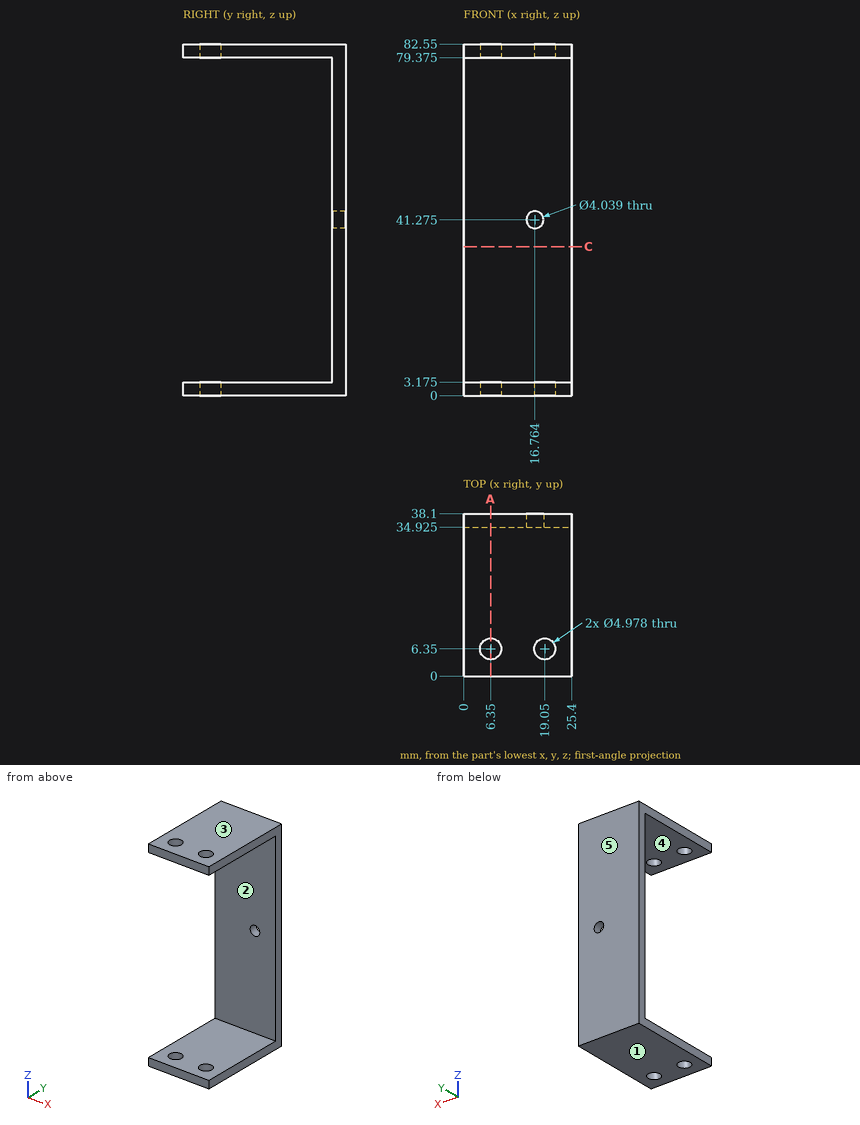
Can you work these out from the drawing? Everything is in mm from the part's minimum corner. A direction names the side the tool comes from. Round coordinates to 2 decimals unless told otherwise and drop trailing zeros. Loops run counter-clockwise (first coordinate to the right, second up) from the corner with the lowest first, then second, coordinate; pieces in that order, holes last. Notation, with made-up numbers: (-24, -19.75) - (19, -19.75) arc R20 cw to (19, 0.25) - close; hole circle Ø8 at (49, 13). An arc over 180 degrees is marked (long way). Write item = value, one per line. Start each with the question number.
(1) If we mould it in two halves opening along Z, with no side actions, what happens to the marked faces 3, 4 and 5? For each: released by +Z, released by -Z, zero draft, split by the parting line, or undercut.
(2) If we section it at C-C (z = 35): Please give me the cut outline in (x, y) (1 decimal).
(3) If we section it at A-A (x = 6.35): Give the number of separate pieces and of enclosed holes in the cut face.
(4) If I drill on probe 1 along X at (y, z) = (6, 80) (1 decimal); probe 2 along Y at (x, z) = (19.05, 81.2); probe 3 along Y at (x, z) = (10, 70) (1 decimal), over which ranges is the centre line in solid material (lowest first)? Write a range as [from, to].
(5) For the marked faces 1 and 2, which set-ups out of +Z, -Z, +X, -X, +Y, -Y let a thin tool reach every point of the face, with its end or its side?
(6) For P1, Ø4, axis at x = 6.35, y = 6.35, coming from the -Z side; P2, Ø6, axis at x = 20.5, z = 49.5, coming from the -Y side (3 decimals), each with a flat end and sliding along its axis, tell me the tip position at first contact or that it passes through.
Ans:
q1.face_3 = released by +Z
q1.face_4 = undercut
q1.face_5 = zero draft
q2.outline = (0, 34.9) - (25.4, 34.9) - (25.4, 38.1) - (0, 38.1) - close
q3.separate_pieces = 3
q3.enclosed_holes = 0
q4.probe_1 = [0, 3.9], [8.8, 16.6], [21.5, 25.4]
q4.probe_2 = [0, 3.86], [8.84, 38.1]
q4.probe_3 = [34.9, 38.1]
q5.face_1 = -Z, +X, -X, +Y, -Y
q5.face_2 = +X, -X, -Y
q6.P1 = through
q6.P2 = 34.925
